from build123d import *

# Parameters (mm, degrees)
F0_W     = 56
F0_H     = 68
F0_R     = 2.25
F1_DEPTH = 12
F2_R     = 4


with BuildPart() as f1:
    # F0 (on Front) → F1 (new body)
    with BuildSketch(Plane.XZ):
        Rectangle(F0_W, F0_H)
        with Locations((-11.5, -11.5)):
            Circle(F0_R, mode=Mode.SUBTRACT)
        with Locations((11.5, -11.5)):
            Circle(F0_R, mode=Mode.SUBTRACT)
        with Locations((-11.5, 11.5)):
            Circle(F0_R, mode=Mode.SUBTRACT)
        with Locations((11.5, 11.5)):
            Circle(F0_R, mode=Mode.SUBTRACT)
    extrude(amount=F1_DEPTH)

    # F2
    f2_edges = [f1.edges().sort_by_distance(p)[0] for p in [
        (28, -6, -34),
        (-28, -6, -34),
        (28, -6, 34),
        (-28, -6, 34),
    ]]
    fillet(f2_edges, radius=F2_R)


solid = f1.part
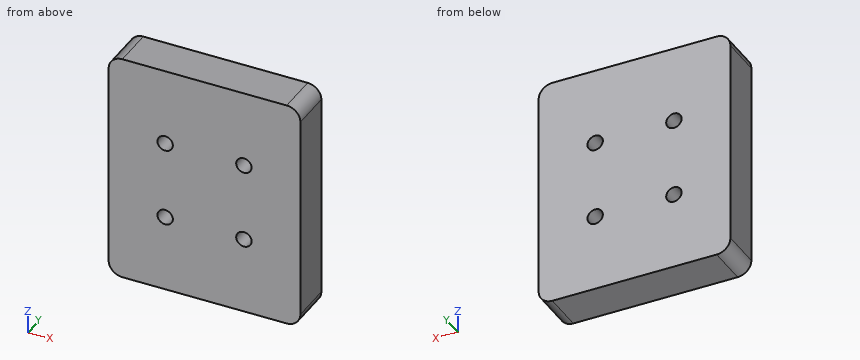
Source: CAD feature listing. Evaluate the final solid. Frame: model axes, mm. Round coordinates to 2 decimals unless told otherwise and drop trailing zeros. Loops run counter-clockwise (first coordinate to the right, second up) from the corner with the lowest first, then second, coordinate; pieces in that order, holes last.
Q1. Ray query, line 1 (Z direction, x = -11.5, y = -8.5); line 2 (Z direction, x = 13, y = -4.5); line 3 (Z direction, x = -25, y = -6.25). Return the intervals inside material, ascending.
Q2. Section B-B, the plane x = -11.5. Return loops of the section in (y, z), plus the area to 3 significant figures.
Q3. Section A-A, the plane z = 11.5. Return loops of the section in (x, y).
Q4. Section C-C, the plane y = -8. Return loops of the section in (x, z).
Solutions:
1. line 1: z = -34 to -13.75, -9.25 to 9.25, 13.75 to 34
1. line 2: z = -34 to -13.18, -9.82 to 9.82, 13.18 to 34
1. line 3: z = -33.87 to 33.87
2. outline: (-12, -34) - (0, -34) - (0, -13.75) - (-12, -13.75) - close; (-12, -9.25) - (0, -9.25) - (0, 9.25) - (-12, 9.25) - close; (-12, 13.75) - (0, 13.75) - (0, 34) - (-12, 34) - close
2. area: 708 mm2
3. outline: (-28, -12) - (-13.75, -12) - (-13.75, 0) - (-28, 0) - close; (-9.25, -12) - (9.25, -12) - (9.25, 0) - (-9.25, 0) - close; (13.75, -12) - (28, -12) - (28, 0) - (13.75, 0) - close
4. outline: (-28, -30) arc R4 ccw to (-24, -34) - (24, -34) arc R4 ccw to (28, -30) - (28, 30) arc R4 ccw to (24, 34) - (-24, 34) arc R4 ccw to (-28, 30) - close; hole circle Ø4.5 at (-11.5, -11.5); hole circle Ø4.5 at (-11.5, 11.5); hole circle Ø4.5 at (11.5, -11.5); hole circle Ø4.5 at (11.5, 11.5)
